The figure shows three views and two pictorial views of one solid part (mm, origin at its lowest corner). Answer the questions. A direction names the side the tool comes from. Round coordinates to 2 decimals unless told otherwise and drop trailing zeros. Write each loop counter-clockwise with the first axis right and the second up, starting at its lowest first coordinate (ties: lowest second). Pieces come first, ordered by that corner, then holes.
Item 1: A tool of negligible diameter and unlimited length cuts with its end or side. For the marked faces 4, 5, 6 and 7, from which of +Z, -Z, +X, -X, +Y, -Y can it reach the whole face along a straight path? Write none if from no direction.
Item 2: Find the intervals of material crossed by probe 1 along Y at (x, z) = (13.75, 1.8); probe 2 along X at (y, z) = (7.5, 2.7); probe 3 along X at (y, z) = (25, 2.6), in increasing order.
Item 3: This flat-tipped pin is pushed along its axis until it touches: pin 1 (8 mm diameter, centred on x = 14, y = 10.5, fed in from -Z). Where does it stop, or does it pass through?
Item 4: Find section A-A on y = 11.5. Give the vertices of the cut face in (x, z).
Item 5: Find section B-B on x = 7.25. Give the vertices of the cut face in (y, z).
Item 6: For a pull along Y with two mould halves and no side action, classify the marked faces 1, 2 and 3 as +Y half, -Y half, draft (parallel to the pull), parting line (faces both ways), or undercut.
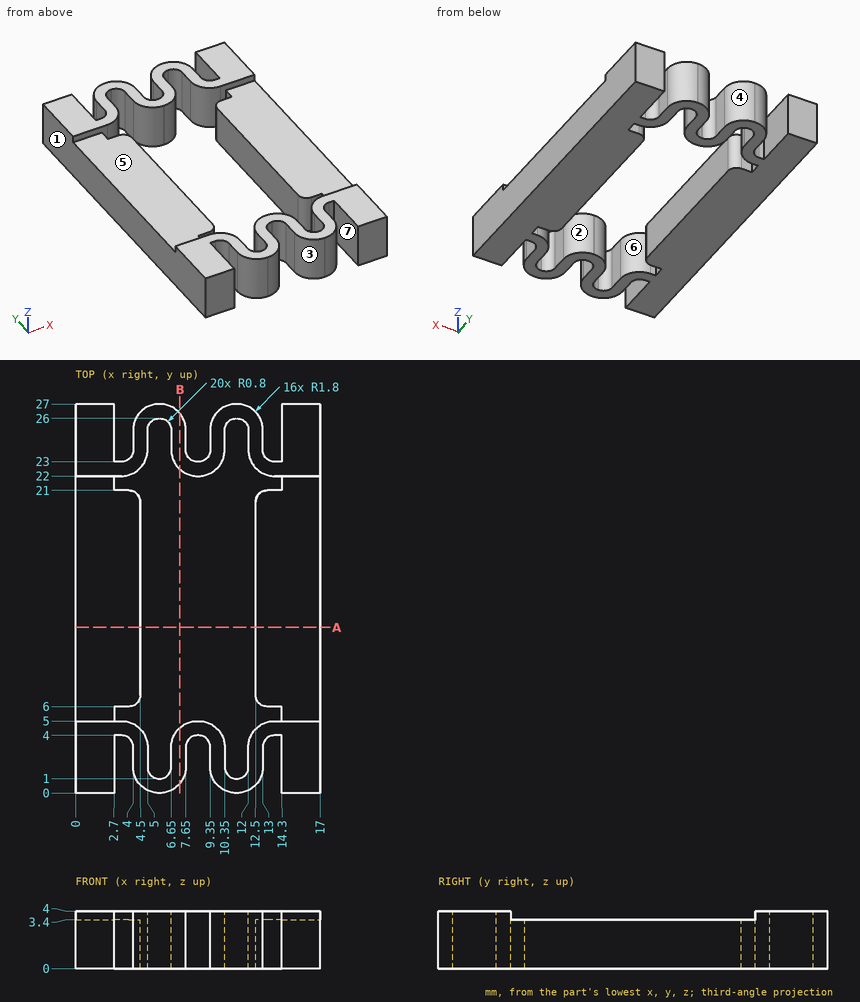
Check values:
1. face 4: +Z, -Z, +Y
1. face 5: +Z, +X, -X
1. face 6: +Z, -Z
1. face 7: +Z, -Z, -Y
2. probe 1: y = 4 to 5, 6 to 21, 22 to 23
2. probe 2: x = 0 to 4.5, 12.5 to 17
2. probe 3: x = 0 to 2.7, 4 to 5, 6.65 to 7.65, 9.35 to 10.35, 12 to 13, 14.3 to 17
3. pin 1: stops at z = 0
4. outline: (0, 0) - (4.5, 0) - (4.5, 3.4) - (0, 3.4) - close; (12.5, 0) - (17, 0) - (17, 3.4) - (12.5, 3.4) - close
5. outline: (0.67, 0) - (4.54, 0) - (4.54, 4) - (0.67, 4) - close; (22.46, 0) - (26.33, 0) - (26.33, 4) - (22.46, 4) - close
6. face 1: draft
6. face 2: undercut
6. face 3: -Y half
